Input: part model. Units: mm. Frame: model coordinates. A direction names the side the tool comes from. Coordinates: 2 decimals unless noted, no trailing zeros. Loops run counter-clockwise (first coordinate to the right, second up) from the corner with the lowest first, then second, coordinate; pieces in that order, holes last.
(1) Contact query for flat-ended pins moving along their axis: P1, Ø4.5, axis at x = -4, y = 1.5, coming from the +Z side; P2, Ø3, axis at x = -5.05, y = 0, coming from the +Z side; P3, Ø3, axis at x = 6, y = -2, coming from the +Z side. Output: stop coordinate, or through.
(2) Section B-B, the plane z = 63. Return loops of the section in (x, y), then the cut area to 3 significant figures.
(3) Line query: L1, parallel to X at y = -3.75, z = 63.75; L2, parallel to Y at x = -5.05, z = 68.9; L3, parallel to Y at x = -5.05, z = 74.2. Output: solid intervals per line, ascending.
(4) Mould query, pull axis X, two halves, no side actions, for faces 1 (the face through (7.95, 0, 63)), 2 (the face through (0, 0, 45)), 3 (the face through (0, 0, 68)). Classes: released by +X, released by -X, zero draft, split by the parting line, or undercut.
(5) Section A-A, the plane x = -5.05. Return loops of the section in (y, z), then the cut area to 3 significant figures.
(6) Section C-C, the plane z = 56.5. Return loops of the section in (x, y), then the cut area to 3 significant figures.
(7) Set-up query: faces 4 (the face through (0, 0, 75)), 5 (the face through (-3.203, -0.766, 57.549)), 6 (the face through (9.75, 0, 66)). Return all of +Z, -Z, +X, -X, +Y, -Y with unobstructed straight access to the full face (end or side cutting, diameter ignored); none if empty.
Autodesk Inventor part; units mm, degrees
ref_plane "YZ Plane" through (0, 0, 0) normal (1, 0, 0) x (0, 1, 0)
ref_plane "XZ Plane" through (0, 0, 0) normal (0, 1, 0) x (-1, 0, 0)
ref_plane "XY Plane" through (0, 0, 0) normal (0, 0, 1) x (1, 0, 0)
sketch "Esquisse1" plane through (0, 0, 0) normal (0, 1, 0) x (-1, 0, 0)
  line L0 (12.8426, 45) -> (-12.8426, 45)
  line L1 (-12.8426, 45) -> (-12.8426, 75)
  line L2 (-12.8426, 75) -> (12.8426, 75)
  line L3 (12.8426, 75) -> (12.8426, 45)
  line L4 (9.75, 67) -> (-9.75, 67)
  line L5 (-9.75, 67) -> (-9.75, 64.2)
  line L6 (-9.75, 64.2) -> (9.75, 64.2)
  line L7 (9.75, 64.2) -> (9.75, 67)
  line L8 (0, -15) -> (0, 90)
  point P0 (0, 0)
  point P1 (0, 64.2)
  point P2 (0, 45)
  dimension "d0" = 75
  dimension "d1" = 19.5
  dimension "d2" = 2.8
  dimension "d3" = 8
  dimension "d45" = 30
  dimension "d46" = 25.6852
extrude "Extrusion1" add sketch "Esquisse1" along normal mid plane 8.2 contours L0 L8 L6 L7 L4 L2 L3 | L0 L1 L2 L8 L4 L5 L6
sketch "Esquisse2" plane through (-12.8426, -4.1, 75) normal (0, 0, 1) x (1, 0, 0)
  circle A0 centre (17.8926, 4.1) radius 3.85
  circle A1 centre (7.7926, 4.1) radius 3.85
  line L0 (17.8926, 4.1) -> (7.7926, 4.1) construction
  line L1 (12.8426, -1.64) -> (12.8426, 9.84) construction
  point P0 (12.8426, 4.1)
  dimension "d6" = 7.7
  dimension "d7" = 10.1
extrude "Extrusion2" cut sketch "Esquisse2" against normal blind 1
sketch "Esquisse3" plane through (-12.8426, -4.1, 74) normal (0, 0, 1) x (1, 0, 0)
  circle A0 centre (7.7926, 4.1) radius 3.85
  circle A1 centre (7.7926, 4.1) radius 2
  circle A2 centre (17.8926, 4.1) radius 3.85
  circle A3 centre (17.8926, 4.1) radius 2
  point P0 (12.8426, 4.1)
  point P1 (9.3965, 7)
  point P2 (9.3965, 0)
  point P3 (16.2887, 0)
  point P4 (16.2887, 7)
  dimension "d10" = 4
  dimension "d11" = 4
extrude "Extrusion3" cut sketch "Esquisse3" against normal blind 20 contours A1 | A3
chamfer "Chanfrein1" distance 1.8 angle 45 2 edges at (-7.05, 0, 74) (3.05, 0, 74)
sketch "Esquisse5" plane through (0, 4.1, 0) normal (0, 1, 0) x (1, 0, 0)
  line L0 (-9.75, -64.2) -> (9.75, -64.2)
  line L1 (-7.95, -64.2) -> (-2.15, -64.2)
  line L2 (-2.15, -64.2) -> (-2.15, -61)
  line L3 (-2.15, -61) -> (-7.95, -61)
  line L4 (-7.95, -61) -> (-7.95, -64.2)
  line L5 (2.15, -64.2) -> (7.95, -64.2)
  line L6 (7.95, -64.2) -> (7.95, -61)
  line L7 (7.95, -61) -> (2.15, -61)
  line L8 (2.15, -61) -> (2.15, -64.2)
  line L9 (5.05, 15) -> (5.05, -90)
  line L10 (-5.05, 15) -> (-5.05, -90)
  line L11 (9.75, -67) -> (-9.75, -67)
  line L12 (-0.6, -67) -> (0.6, -67)
  line L13 (0.6, -67) -> (0.6, -68)
  line L14 (0.6, -68) -> (-0.6, -68)
  line L15 (-0.6, -68) -> (-0.6, -67)
  point P0 (0, 0)
  point P1 (5.05, -64.2)
  point P2 (-5.05, -64.2)
  point P3 (0, -67)
  dimension "d17" = 5.8
  dimension "d18" = 3.2
  dimension "d19" = 3.2
  dimension "d22" = 1.2
  dimension "d24" = 1
extrude "Extrusion4" cut sketch "Esquisse5" against normal blind 20 contours L0 L10 L3 L2 | L8 L7 L9 L0 | L0 L4 L3 L10 | L9 L7 L6 L0 | L11 L13 L14 L15
properties part number "base1"
Report:
1. P1: stops at z = 75
1. P2: stops at z = 54
1. P3: stops at z = 73.91
2. outline: (-12.84, -4.1) - (-7.95, -4.1) - (-7.95, 4.1) - (-12.84, 4.1) - close; (-2.15, -4.1) - (2.15, -4.1) - (2.15, 4.1) - (-2.15, 4.1) - close; (7.95, -4.1) - (12.84, -4.1) - (12.84, 4.1) - (7.95, 4.1) - close
2. area: 115 mm2
3. L1: x = -12.84 to -7.95, -2.15 to 2.15, 7.95 to 12.84
3. L2: y = -4.1 to -2, 2 to 4.1
3. L3: y = -4.1 to -3.85, 3.85 to 4.1
4. face 1: undercut
4. face 2: zero draft
4. face 3: undercut
5. outline: (-4.1, 45) - (4.1, 45) - (4.1, 61) - (2, 61) - (2, 54) - (-2, 54) - (-2, 61) - (-4.1, 61) - close; (-4.1, 67) - (-2, 67) - (-2, 72.2) - (-3.8, 74) - (-3.85, 74) - (-3.85, 75) - (-4.1, 75) - close; (2, 67) - (4.1, 67) - (4.1, 75) - (3.85, 75) - (3.85, 74) - (3.8, 74) - (2, 72.2) - close
5. area: 130 mm2
6. outline: (-12.84, -4.1) - (12.84, -4.1) - (12.84, 4.1) - (-12.84, 4.1) - close; hole circle Ø4 at (-5.05, 0); hole circle Ø4 at (5.05, 0)
6. area: 185 mm2
7. face 4: +Z, +X, -X, +Y, -Y
7. face 5: +Z
7. face 6: +Y, -Y
